Verification items for the finished model (mm, model axes). A direction names the side the tool comes from. Coordinates: 2 decimals unless noted, no trailing zeros. Write each loop counter-clockwise with the first axis right and the second up, starting at its lowest first coordinate (ties: lowest second). Pieces come first, ordered by that corner, then holes. Notation, with made-up numbers: M 17,72 L 69,72 A16 cw 69,80 Z; hole C 71.25,-2 d8. An arc over 180 degrees is marked long. Answer in a Markdown table with one row per item.
from build123d import *

# Parameters (mm, degrees)
POCKET_DEPTH = 5
FILLET_R     = 1
FILLET001_R  = 1
FILLET002_R  = 1


with BuildPart() as part:
    # Sketch → Revolution (revolve)
    with BuildSketch(Plane.YZ):
        Polygon((0, 0), (14.142, 0), (14.142, 5.4), (10.683, 5.4), (8.165701, 2.4), (0, 2.4), align=None)
    revolve(axis=Axis((0, 0, 0), (0, 0, 1)))

    # Sketch001 (on Face5 of Revolution) → Pocket (cut)
    with BuildSketch(Plane(origin=(0, 0, 2.4), x_dir=(0, -1, 0), z_dir=(0, 0, 1))):
        with BuildLine():
            Line((-5, 2.6), (5, 2.6))
            ThreePointArc((5, -2.6), (7.6, 0), (5, 2.6))
            Line((-5, -2.6), (5, -2.6))
            ThreePointArc((-5, 2.6), (-7.6, 0), (-5, -2.6))
        make_face()
    extrude(amount=-POCKET_DEPTH, mode=Mode.SUBTRACT)

    # Fillet
    fillet_edges = [part.edges().sort_by_distance(p)[0] for p in [
        (0, -8.165701, 2.4),
    ]]
    fillet(fillet_edges, radius=FILLET_R)

    # Fillet001
    fillet001_edges = [part.edges().sort_by_distance(p)[0] for p in [
        (0, 7.6, 2.4),
    ]]
    fillet(fillet001_edges, radius=FILLET001_R)

    # Fillet002
    fillet002_edges = [part.edges().sort_by_distance(p)[0] for p in [
        (0, -10.683, 5.4),
    ]]
    fillet(fillet002_edges, radius=FILLET002_R)


solid = part.part
1) Sectioned sample at C-C (z = 4.6). Record the cut outline in (x, y).
Response values:
| item | result |
|---|---|
| outline | C 0,0 d28.28; hole C 0,0 d20.02 |
2) Sectioned sample at B-B (z = 0.7). Record the cut outline in (x, y).
Response values:
| item | result |
|---|---|
| outline | C 0,0 d28.28; hole M -2.6,-5 A2.6 ccw 2.6,-5 L 2.6,5 A2.6 ccw -2.6,5 Z |
3) Release check for a two-part mould opening along Y. For faces 4 (the face through (-0.1, -7.6, 0.7)), 5 (the face through (-5, 0, 2.4)), 6 (the face through (4, -11, 5.4)), 7 (the face through (8.61, -11.22, 2.74)) record: +Y half, -Y half, draft (parallel to the pull), parting line (faces both ways), or undercut.
Response values:
| item | result |
|---|---|
| face 4 | undercut |
| face 5 | undercut |
| face 6 | draft |
| face 7 | parting line |
4) Depth check by flat-ended pin: pin 1 (1.5 mm diameter, centred on x = -8, z = 1, fed in from -Y); pin 2 (2.5 mm diameter, centred on x = 4.5, y = -1, fed in from +Z); pin 3 (1.5 mm diameter, centred on y = 2.5, z = 1, fed in from +X); pin 4 (3 mm diameter, centred on x = -10, y = -10.5, fed in from -Z). Enter the tip coordinate at first touch or a pass-through.
Response values:
| item | result |
|---|---|
| pin 1 | stops at y = -12.14 |
| pin 2 | stops at z = 2.4 |
| pin 3 | stops at x = 14.03 |
| pin 4 | stops at z = 0 |
5) Sectioned sample at A-A (y = 0). Record the cut outline in (x, z), then the cut area to 3 significant figures.
Response values:
| item | result |
|---|---|
| outline | M -14.14,0 L -2.6,0 L -2.6,1.4 A1 ccw -3.6,2.4 L -7.7,2.4 A1 cw -8.47,2.76 L -10.38,5.04 A1 ccw -11.15,5.4 L -14.14,5.4 Z; M 2.6,0 L 14.14,0 L 14.14,5.4 L 11.15,5.4 A1 ccw 10.38,5.04 L 8.47,2.76 A1 cw 7.7,2.4 L 3.6,2.4 A1 ccw 2.6,1.4 Z |
| area | 83.3 mm² |
6) Thickness scan on L1, parallel to Y at x = -8.25, z = 5.15; L2, parallel to X at y = 4.5, z = 4; L3, parallel to X at y = -5.5, z = 2.75. Record the ranges inside material, lowest first. Write a range as [from, to].
Response values:
| item | result |
|---|---|
| L1 | y = [-11.49, -6.48], [6.48, 11.49] |
| L2 | x = [-13.41, -8.38], [8.38, 13.41] |
| L3 | x = [-13.03, -6.43], [6.43, 13.03] |
7) Tool access check on faces 1 (the face through (3, 0, 0)), 2 (the face through (5, 0, 2.4)), 3 (the face through (-2.6, 0, 1)). Record the directions out of +Z, -Z, +X, -X, +Y, -Y that give a thin tool (end or side, any length) a straight path to the whole face; none if there is none.
Response values:
| item | result |
|---|---|
| face 1 | -Z, +X, -X, +Y, -Y |
| face 2 | +Z |
| face 3 | +Z, -Z |
